The listing builds one solid part. Answer for the finished solid, in the listing's coordinates (mm). A direction names the side the tool comes from. Give positions to 0.01 mm unless a question says otherwise; leave off trailing zeros. Order: outer loops, then holes, each group sorted by start corner. A loop starts at its lowest first (then second) coordinate and runs counter-clockwise, first axis right, second up. Notation, with made-up numbers: (30, -23.5) -> (64, -23.5) arc R23 cw to (64, -12.5) -> close; hole circle Ø1 at (61, 42). An arc over 180 degrees is marked (long way). Answer as a JSON object with one key per item and string values. Group by question number.
```python
from build123d import *

# Parameters (mm, degrees)
SKETCH1_R           = 2.585044133
BOSS_EXTRUDE1_DEPTH = 7.62


with BuildPart() as part:
    # Sketch1 → Boss-Extrude1 (new body)
    with BuildSketch(Plane(origin=(0, 0, 0), x_dir=(1, 0, 0), z_dir=(0, 1, 0))):
        with BuildLine():
            Line((3.020276381, 31.156144465), (1.399779997, 30.876318364))
            Line((1.399779997, 30.876318364), (-10.128325028, 14.535897116))
            Line((-10.128325028, 14.535897116), (-8.192029601, 3.322648137))
            ThreePointArc((-8.192029601, 3.322648137), (-18.968565906, -37.532030496), (4.88487987, -72.406829787))
            Line((4.88487987, -72.406829787), (-3.568924444, -73.866626378))
            ThreePointArc((-3.568924444, -73.866626378), (-27.113440564, -40.443559332), (-18.408519275, -0.497721057))
            Line((-18.408519275, -0.497721057), (-17.051314308, 4.21102278))
            Line((-17.051314308, 4.21102278), (-18.796078997, 14.315101218))
            Line((-18.796078997, 14.315101218), (-2.622690692, 37.239942495))
            Line((-2.622690692, 37.239942495), (1.836758298, 38.009996803))
            ThreePointArc((1.836758298, 38.009996803), (1.726185886, 38.158240643), (1.62669315, 38.31413705))
            ThreePointArc((1.62669315, 38.31413705), (1.699886001, 38.484843232), (1.777492058, 38.653588881))
            ThreePointArc((1.777492058, 38.653588881), (2.738177728, 38.665878668), (3.634702712, 38.320464496))
            ThreePointArc((3.634702712, 38.320464496), (3.859539856, 38.666818829), (4.110435884, 38.994788717))
            ThreePointArc((4.110435884, 38.994788717), (3.484366991, 39.723558733), (3.173770753, 40.632733069))
            ThreePointArc((3.173770753, 40.632733069), (3.306718558, 40.762435326), (3.44299337, 40.888637424))
            ThreePointArc((3.44299337, 40.888637424), (4.335254295, 40.532353217), (5.031351097, 39.870146876))
            ThreePointArc((5.031351097, 39.870146876), (5.371617597, 40.104095105), (5.728923946, 40.311086019))
            ThreePointArc((5.728923946, 40.311086019), (5.42939992, 41.223967914), (5.490372369, 42.182795508))
            ThreePointArc((5.490372369, 42.182795508), (5.662835029, 42.251747846), (5.837031991, 42.316193269))
            ThreePointArc((5.837031991, 42.316193269), (6.525029535, 41.645576109), (6.914723727, 40.767392511))
            ThreePointArc((6.914723727, 40.767392511), (7.318617093, 40.853318139), (7.727937109, 40.907817588))
            ThreePointArc((7.727937109, 40.907817588), (7.800557769, 41.865833368), (8.223816402, 42.728341412))
            ThreePointArc((8.223816402, 42.728341412), (8.409538041, 42.726046463), (8.595137244, 42.718923979))
            ThreePointArc((8.595137244, 42.718923979), (8.974130017, 41.836069249), (8.998094191, 40.875603886))
            ThreePointArc((8.998094191, 40.875603886), (9.40412532, 40.800425515), (9.803143741, 40.694136452))
            ThreePointArc((9.803143741, 40.694136452), (10.236853249, 41.5514369), (10.957960776, 42.186316362))
            ThreePointArc((10.957960776, 42.186316362), (11.128666958, 42.113123511), (11.297412607, 42.035517454))
            ThreePointArc((11.297412607, 42.035517454), (11.309702393, 41.074831784), (10.964288222, 40.1783068))
            ThreePointArc((10.964288222, 40.1783068), (11.310642554, 39.953469656), (11.638612443, 39.702573628))
            ThreePointArc((11.638612443, 39.702573628), (12.367382459, 40.328642521), (13.276556795, 40.639238759))
            ThreePointArc((13.276556795, 40.639238759), (13.406259052, 40.506290954), (13.53246115, 40.370016142))
            ThreePointArc((13.53246115, 40.370016142), (13.176176943, 39.477755216), (12.513970602, 38.781658415))
            ThreePointArc((12.513970602, 38.781658415), (12.747918831, 38.441391914), (12.954909744, 38.084085566))
            ThreePointArc((12.954909744, 38.084085566), (13.867791639, 38.383609592), (14.826619234, 38.322637143))
            ThreePointArc((14.826619234, 38.322637143), (14.895571572, 38.150174482), (14.960016995, 37.975977521))
            ThreePointArc((14.960016995, 37.975977521), (14.289399835, 37.287979977), (13.411216236, 36.898285785))
            ThreePointArc((13.411216236, 36.898285785), (13.497141864, 36.494392418), (13.551641313, 36.085072403))
            ThreePointArc((13.551641313, 36.085072403), (14.509657094, 36.012451743), (15.372165138, 35.58919311))
            ThreePointArc((15.372165138, 35.58919311), (15.369870189, 35.403471471), (15.362747705, 35.217872267))
            ThreePointArc((15.362747705, 35.217872267), (14.479892975, 34.838879495), (13.519427611, 34.814915321))
            ThreePointArc((13.519427611, 34.814915321), (13.444249241, 34.408884192), (13.337960178, 34.009865771))
            ThreePointArc((13.337960178, 34.009865771), (14.195260626, 33.576156263), (14.830140088, 32.855048736))
            ThreePointArc((14.830140088, 32.855048736), (14.756947237, 32.684342554), (14.67934118, 32.515596905))
            ThreePointArc((14.67934118, 32.515596905), (13.718655509, 32.503307119), (12.822130526, 32.84872129))
            ThreePointArc((12.822130526, 32.84872129), (12.597293382, 32.502366958), (12.346397354, 32.174397069))
            ThreePointArc((12.346397354, 32.174397069), (12.972466247, 31.445627053), (13.283062484, 30.536452717))
            ThreePointArc((13.283062484, 30.536452717), (13.15011468, 30.40675046), (13.013839868, 30.280548362))
            ThreePointArc((13.013839868, 30.280548362), (12.121578942, 30.636832569), (11.42548214, 31.29903891))
            ThreePointArc((11.42548214, 31.29903891), (11.08521564, 31.065090681), (10.727909292, 30.858099767))
            ThreePointArc((10.727909292, 30.858099767), (11.027433317, 29.945217873), (10.966460868, 28.986390278))
            ThreePointArc((10.966460868, 28.986390278), (10.793998208, 28.91743794), (10.619801246, 28.852992517))
            ThreePointArc((10.619801246, 28.852992517), (9.931803703, 29.523609677), (9.54210951, 30.401793275))
            ThreePointArc((9.54210951, 30.401793275), (9.138216144, 30.315867647), (8.728896129, 30.261368198))
            ThreePointArc((8.728896129, 30.261368198), (8.656275469, 29.303352418), (8.233016836, 28.440844374))
            ThreePointArc((8.233016836, 28.440844374), (8.047295197, 28.443139323), (7.861695993, 28.450261807))
            ThreePointArc((7.861695993, 28.450261807), (7.482703221, 29.333116537), (7.458739046, 30.2935819))
            ThreePointArc((7.458739046, 30.2935819), (7.052707918, 30.368760271), (6.653689497, 30.475049334))
            ThreePointArc((6.653689497, 30.475049334), (6.219979988, 29.617748886), (5.498872462, 28.982869424))
            ThreePointArc((5.498872462, 28.982869424), (5.32816628, 29.056062275), (5.159420631, 29.133668332))
            ThreePointArc((5.159420631, 29.133668332), (5.147130844, 30.094354002), (5.492545016, 30.990878986))
            ThreePointArc((5.492545016, 30.990878986), (5.146190683, 31.21571613), (4.818220795, 31.466612158))
            ThreePointArc((4.818220795, 31.466612158), (4.089450779, 30.840543265), (3.180276443, 30.529947028))
            ThreePointArc((3.180276443, 30.529947028), (3.050574186, 30.662894832), (2.924372087, 30.799169644))
            ThreePointArc((2.924372087, 30.799169644), (2.965822028, 30.979403927), (3.020276381, 31.156144465))
        make_face()
        with Locations(Location((8.228416619, 35.584592893, 0), (0, 0, 90))):
            Circle(SKETCH1_R, mode=Mode.SUBTRACT)
    extrude(amount=BOSS_EXTRUDE1_DEPTH)


solid = part.part
```
(1) For a pull along X with two mould halves and no side action, classify faces 1 (the cylindrical face through (-26.993, 3.757, 41.02)), 2 (the cylindrical face through (13.85, 3.76, -38.38)), 3 (the flat face through (0.717, 3.757, 73.127)) as +X half, -X half, draft (parallel to the pull), parting line (faces both ways), or undercut.
(2) A cutting plane is placed at A-A (x = -0.5). Determine the outline of the cut face in (y, z).
(3) Which of the six approach directions +Z, -Z, +X, -X, +Y, -Y give full straight-line access (tool end or side, diameter ignored) to faces 4 (the flat face through (-19, 7.62, 15)), 5 (the flat face through (-19, 0, 15)), 6 (the cylindrical face through (11.026, 3.757, -29.959)), 7 (the flat face through (-9.174, 3.757, -9.008)), 8 (the flat face through (-17.91, 3.76, -9.19))?
(4) A cutting plane is placed at C-C (x = -23). Determine the outline of the cut face in (y, z), and give its area (3 significant figures).
(5) Find the intervals of material crossed by line 1 along Z through (x, y) = (13, 5); line 2 along Z through (x, y) = (-15, 4.5); line 3 along Z through (x, y) = (-5.5, 7.25), in increasing order. Write a range as [from, to].
(6) A cutting plane is placed at B-B (z = -20). Determine the outline of the cut face in (x, y).
(7) Flat-ended cylindrical pins translate along their axes: pin 1 Ø2 at (y, z) = (1.5, 42) entering from +X; pin 2 Ø4 at (x, z) = (8.23, -35.58) entering from -Y; pin 3 Ø4 at (y, z) = (7, 40) entering from +X; pin 4 Ø3 at (x, y) = (-16, 2.5) entering from +Z. Find the tip coordinate at first contact, or state that the pin passes through.
Check sheet entries:
{
 "1": {"face 1": "-X half", "face 2": "undercut", "face 3": "+X half"},
 "2": {"outline": "(0, -37.61) -> (7.62, -37.61) -> (7.62, -28.18) -> (0, -28.18) -> close; (0, 68.67) -> (7.62, 68.67) -> (7.62, 73.34) -> (0, 73.34) -> close"},
 "3": {"face 4": "+Z, -Z, +X, -X, +Y", "face 5": "+Z, -Z, +X, -X, -Y", "face 6": "+Y, -Y", "face 7": "+X, +Y, -Y", "face 8": "-X, +Y, -Y"},
 "4": {"outline": "(0, 8.14) -> (7.62, 8.14) -> (7.62, 52.6) -> (0, 52.6) -> close", "area": "339 mm2"},
 "5": {"line 1": "z = [-40.58, -39.24], [-38.11, -32.75], [-31.4, -30.28]", "line 2": "z = [-19.7, 7.53], [50.25, 64.45]", "line 3": "z = [-33.16, -21.1], [64.13, 72.64]"},
 "6": {"outline": "(-14.79, 0) -> (-6.27, 0) -> (-6.27, 7.62) -> (-14.79, 7.62) -> close"},
 "7": {"pin 1": "stops at x = -17.71", "pin 2": "passes through", "pin 3": "stops at x = -17.99", "pin 4": "stops at z = 64.99"}
}
